Build history of the part. All positions in model axes, mm. A direction names the side the tool comes from. Round coordinates to 2 decimals unless told otherwise and drop trailing zeros. Write each loop counter-clockwise with the first axis right and the second up, starting at its lowest first coordinate (ties: lowest second). Pieces come first, ordered by that corner, then holes. Notation, with made-up numbers: M -32,64 L -12,64 A21 cw -12,100 Z; hole C 55.5,-35.75 d11. An arc over 180 degrees is marked long. Use a Markdown table: item, result.
Autodesk Inventor part; units mm, degrees
ref_plane "YZ Plane" through (0, 0, 0) normal (1, 0, 0) x (0, 1, 0)
ref_plane "XZ Plane" through (0, 0, 0) normal (0, 1, 0) x (-1, 0, 0)
ref_plane "XY Plane" through (0, 0, 0) normal (0, 0, 1) x (1, 0, 0)
sketch "Sketch1" plane through (0, 0, 0) normal (0, 0, 1) x (1, 0, 0)
  line L0 (-22.5, 22.5) -> (-6, 22.5)
  line L1 (-6, 22.5) -> (-6, 21)
  line L2 (-6, 21) -> (-5, 21)
  line L3 (-5, 21) -> (-5, 16.5)
  line L4 (-5, 16.5) -> (-10, 16.5)
  line L5 (-10, 16.5) -> (-10, 12.5)
  line L6 (-10, 12.5) -> (-5, 10)
  line L7 (-5, 10) -> (5, 10)
  line L8 (10, 12.5) -> (10, 16.5)
  line L9 (10, 16.5) -> (5, 16.5)
  line L10 (5, 16.5) -> (5, 21)
  line L11 (5, 21) -> (6, 21)
  line L12 (6, 21) -> (6, 22.5)
  line L13 (6, 22.5) -> (22.5, 22.5)
  line L14 (22.5, 22.5) -> (22.5, 6)
  line L15 (22.5, 6) -> (21, 6)
  line L16 (21, 6) -> (21, 5)
  line L17 (21, 5) -> (16.5, 5)
  line L18 (10, 12.5) -> (5, 10)
  line L19 (-22.5, 0) -> (-22.5, 104.1484) construction
  line L20 (-22.5, 0) -> (77.4828, 0) construction
  line L21 (16.5, 5) -> (16.5, 10)
  line L22 (16.5, 10) -> (12.5, 10)
  line L23 (12.5, 10) -> (10, 5)
  line L24 (10, 5) -> (10, 0)
  circle A0 centre (0, 0) radius 6
  circle A1 centre (16.5, 16.5) radius 3
  line L25 (-22.5, 0) -> (45.512, 0) construction
  line L26 (21, -6) -> (21, -5)
  line L27 (22.5, -6) -> (21, -6)
  line L28 (10, -12.5) -> (10, -16.5)
  line L29 (12.5, -10) -> (10, -5)
  line L30 (16.5, -5) -> (16.5, -10)
  line L31 (16.5, -10) -> (12.5, -10)
  line L32 (10, -12.5) -> (5, -10)
  line L33 (22.5, -22.5) -> (22.5, -6)
  circle A2 centre (16.5, -16.5) radius 3
  line L34 (6, -22.5) -> (22.5, -22.5)
  line L35 (5, -16.5) -> (5, -21)
  line L36 (5, -21) -> (6, -21)
  line L37 (6, -21) -> (6, -22.5)
  line L38 (10, -16.5) -> (5, -16.5)
  line L39 (21, -5) -> (16.5, -5)
  line L40 (10, -5) -> (10, 0)
  line L41 (-5, -10) -> (5, -10)
  line L42 (-22.5, -22.5) -> (-6, -22.5)
  line L43 (-6, -22.5) -> (-6, -21)
  line L44 (-6, -21) -> (-5, -21)
  line L45 (-5, -21) -> (-5, -16.5)
  line L46 (-5, -16.5) -> (-10, -16.5)
  line L47 (-10, -16.5) -> (-10, -12.5)
  line L48 (-10, -12.5) -> (-5, -10)
  line L49 (-22.5, -22.5) -> (-22.5, 22.5)
  line L50 (0, -24.7031) -> (0, 16.5) construction
  line L51 (-12.5, 10) -> (-10, 5)
  line L52 (-16.5, 10) -> (-12.5, 10)
  line L53 (-16.5, 5) -> (-16.5, 10)
  line L54 (-21, 5) -> (-16.5, 5)
  line L55 (-21, 6) -> (-21, 5)
  line L56 (-22.5, 6) -> (-21, 6)
  line L57 (-10, 5) -> (-10, 0)
  line L58 (-10, -5) -> (-10, 0)
  line L59 (-12.5, -10) -> (-10, -5)
  line L60 (-16.5, -10) -> (-12.5, -10)
  line L61 (-16.5, -5) -> (-16.5, -10)
  line L62 (-21, -5) -> (-16.5, -5)
  line L63 (-21, -6) -> (-21, -5)
  line L64 (-22.5, -6) -> (-21, -6)
  circle A3 centre (-16.5, 16.5) radius 3
  circle A4 centre (-16.5, -16.5) radius 3
  point P0 (0, 10)
  point P1 (0, -10)
  point P2 (-69.7014, -56.3955)
  point P3 (-69.7014, -68.3955)
  point P4 (-36.78, -20.9511)
  point P5 (-36.78, -32.9511)
  dimension "d0" = 22.5
  dimension "d1" = 20
  dimension "d2" = 1.5
  dimension "d3" = 1.5
  dimension "d4" = 10
  dimension "d5" = 12
  dimension "d6" = 12.5
  dimension "d7" = 22.5
  dimension "d8" = 5
  dimension "d9" = 6
  dimension "d10" = 10
  dimension "d11" = 6
  dimension "d12" = 4
  dimension "d13" = 5
  dimension "d14" = 6
  dimension "d15" = 45
  dimension "d16" = 10
  dimension "d17" = 4
  dimension "d18" = 12.5
  dimension "d19" = 6
  dimension "d20" = 12
  dimension "d21" = 22.5
  dimension "d22" = 6
  dimension "d23" = 39
  dimension "d24" = 16.5
  dimension "d25" = 12.5
extrude "Extrusion1" add sketch "Sketch1" along normal mid plane 560 contours L0 L1 L2 L3 L4 L5 L6 L7 L18 L8 L9 L10 L11 L12 L13 L14 L15 L16 L17 L21 L22 L23 L24 L40 L29 L31 L30 L39 L26 L27 L33 L34 L37 L36 L35 L38 L28 L32 L41 L48 L47 L46 L45 L44 L43 L42 L49 L64 L63 L62 L61 L60 L59 L58 L57 L51 L52 L53 L54 L55 L56
equation "\"d3\" = d2"
equation "\"d13\" = d8"
equation "\"d14\" = d9"
equation "\"d16\" = d10"
equation "\"d17\" = d12"
equation "\"d19\" = d11"
properties part number "Union soporte P45X45 Trigger" material "Aluminum 6061"
Q1. Cut at A-A on x = 0. Give the cut face in (y, z).
Response values:
| item | result |
|---|---|
| outline | M -10,-280 L -6,-280 L -6,280 L -10,280 Z; M 6,-280 L 10,-280 L 10,280 L 6,280 Z |
Q2. Drop flat-ended pins along their axis: P1, Ø2, axis at y = 2.5, z = -47, coming from the -X side; P2, Ø0.5, axis at y = 5.5, z = -111.5, coming from the -X side; P3, Ø8, axis at y = -1.5, z = -66.5, coming from the +X side. Give the stop position or say it passes through.
Response values:
| item | result |
|---|---|
| P1 | stops at x = -10 |
| P2 | stops at x = -21 |
| P3 | stops at x = 21 |
Q3. Which spindle directions (+Z, -Z, +X, -X, +Y, -Y) get a long thin tool onto all of the face, cutting with end or side? Do faces 1 (the flat face through (0, -10, -4)), 2 (the flat face through (0, 10, -4)), 3 (the flat face through (-14, 22.5, -4)), 4 (the flat face through (-10, 0, -4)), 5 (the flat face through (10, 0, -4)). Say none if no direction does.
Response values:
| item | result |
|---|---|
| face 1 | +Z, -Z, -Y |
| face 2 | +Z, -Z, +Y |
| face 3 | +Z, -Z, +X, -X, +Y |
| face 4 | +Z, -Z, -X |
| face 5 | +Z, -Z, +X |
Q4. Drill centre lines: L1, parallel to X at y = -16, z = -73; L2, parallel to Y at x = 0, z = -121; L3, parallel to X at y = 0.5, z = -237.5. Where is each one in solid material? Low to high.
Response values:
| item | result |
|---|---|
| L1 | x = -22.5 to -19.46, -13.54 to -10, 10 to 13.54, 19.46 to 22.5 |
| L2 | y = -10 to -6, 6 to 10 |
| L3 | x = -10 to -5.98, 5.98 to 10 |
Q5. Cut at C-C on z = 224.5. Count the separate pieces of the cut face and the enclosed holes in it, and give its area (3 significant figures).
Response values:
| item | result |
|---|---|
| separate pieces | 1 |
| enclosed holes | 5 |
| area | 1,080 mm2 |
Q6. Two-plate mould, pull along Y, no slides. Class faces 6 (the flat face through (14, 22.5, -4)), 7 (the cylindrical face through (-6, 0, -4)), 8 (the flat face through (-22.5, 14, -4)): +Y half, -Y half, draft (parallel to the pull), parting line (faces both ways), or undercut.
Response values:
| item | result |
|---|---|
| face 6 | +Y half |
| face 7 | undercut |
| face 8 | draft |
